Work out the finished part from the listing and answer in its coordinate system (mm). Face numbers are marked on the shaded views. A direction names the side the tool comes from. Round coordinates to 2 decimals unless told otherwise and drop trailing zeros. Write each loop counter-clockwise with the first axis right and the second up, starting at its lowest first coordinate (ties: lowest second). Pieces come first, ordered by that corner, then holes. Notation, with made-up numbers: (-8, 85) -> (42, 85) arc R29 ccw to (42, 123) -> close; hole circle Ø10 at (80, 49.5). An arc over 180 degrees is marked (long way). One line per item, written item: value.
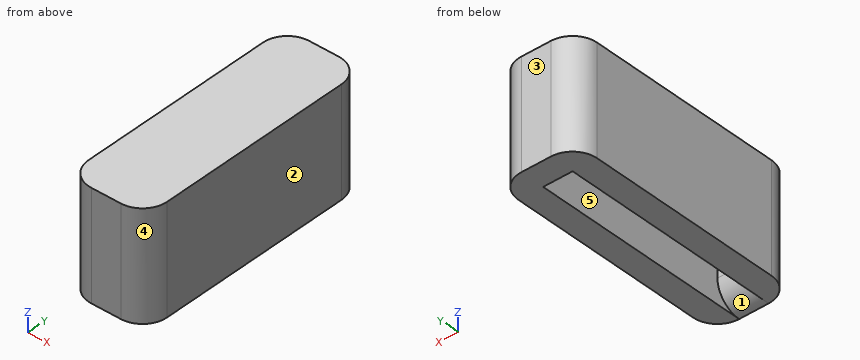
```python
from build123d import *

# Parameters (mm, degrees)
F0_W     = 16
F0_H     = 50
F0_W_2   = 6
F0_H_2   = 40
F1_DEPTH = 12
F2_W     = 16
F2_H     = 50
F3_DEPTH = 10
F4_R     = 4.99999
F5_R     = 5


# Not quite as in the source:
# - a fillet or chamfer is up to 0.001 mm smaller than in the source, because OpenCascade refuses the exact size


with BuildPart() as f1:
    # F0 (on Top) → F1 (new body)
    with BuildSketch(Plane.XY):
        with Locations((-23.0457014143, -5.7597834617)):
            Rectangle(F0_W, F0_H)
        with Locations((-23.0457014143, -5.7597834617)):
            Rectangle(F0_W_2, F0_H_2, mode=Mode.SUBTRACT)
    extrude(amount=F1_DEPTH)

    # F2 (on face) → F3 (join)
    with BuildSketch(Plane.XY.offset(12)):
        with Locations((-23.0457014143, -5.7597834617)):
            Rectangle(F2_W, F2_H)
    extrude(amount=F3_DEPTH)

    # F4 (radius 5 in the source; OpenCascade refuses exactly that, so slightly less here)
    f4_edges = [f1.edges().sort_by_distance(p)[0] for p in [
        (-23.045701, -25.759783, 0),
    ]]
    fillet(f4_edges, radius=F4_R)

    # F5
    f5_edges = [f1.edges().sort_by_distance(p)[0] for p in [
        (-15.045701, 19.240217, 11),
        (-15.045701, -30.759783, 11),
        (-31.045701, -30.759783, 11),
        (-31.045701, 19.240217, 11),
    ]]
    fillet(f5_edges, radius=F5_R)


solid = f1.part
```
(1) Find section D-D on y = -22. Give the vertices of the cut face in (x, z), plus the area to 3 significant figures.
Reported:
outline: (-31.05, 0) -> (-26.05, 0) -> (-26.05, 12) -> (-20.05, 12) -> (-20.05, 0) -> (-15.05, 0) -> (-15.05, 22) -> (-31.05, 22) -> close
area: 280 mm2
(2) Consider probe 1 along X at (y, z) = (14, 9.25); probe 2 along Y at (x, z) = (-23, 11.5); probe 3 along Z at (x, y) = (-22.25, 13.5). Determine where each line is inside the solid, lowest interval first.
Reported:
probe 1: x = -31.05 to -26.05, -20.05 to -15.05
probe 2: y = -30.76 to -25.76, 14.24 to 19.24
probe 3: z = 12 to 22
(3) Find section B-B on z = 15.5. Give the vertices of the cut face in (x, y), plus the area to 3 significant figures.
Reported:
outline: (-31.05, -25.76) arc R5 ccw to (-26.05, -30.76) -> (-20.05, -30.76) arc R5 ccw to (-15.05, -25.76) -> (-15.05, 14.24) arc R5 ccw to (-20.05, 19.24) -> (-26.05, 19.24) arc R5 ccw to (-31.05, 14.24) -> close
area: 779 mm2
(4) A tool of negligible diameter and unlimited length cuts with its end or side. For the marked faces 1 and 2, from which of +Z, -Z, +X, -X, +Y, -Y can it reach the whole face along a straight path? Write none if from no direction.
Reported:
face 1: -Z
face 2: +Z, -Z, +X, +Y, -Y
(5) Find section C-C on z = 9.5. Give the vertices of the cut face in (x, y), plus the area to 3 significant figures.
Reported:
outline: (-31.05, -25.76) arc R5 ccw to (-26.05, -30.76) -> (-20.05, -30.76) arc R5 ccw to (-15.05, -25.76) -> (-15.05, 14.24) arc R5 ccw to (-20.05, 19.24) -> (-26.05, 19.24) arc R5 ccw to (-31.05, 14.24) -> close; hole (-26.05, -25.76) -> (-20.05, -25.76) -> (-20.05, 14.24) -> (-26.05, 14.24) -> close
area: 539 mm2
(6) A flat-ended cylindrical pin translates along its axis: pin 1 Ø1.5 at (x, y) = (-24.5, 6.5) entering from -Z. Find the tip coordinate at first contact, or state that the pin passes through.
Reported:
pin 1: stops at z = 12
(7) For a pull along X with two mould halves and no side action, classify the marked faces 3, 4 and 5 as pulls with the +X half, pulls with the -X half, needs draft (parallel to the pull), parting line crosses it, or undercut.
Reported:
face 3: needs draft
face 4: pulls with the +X half
face 5: undercut
